Here's how the part is built. I have some questions about the finished solid (model axes, mm). Round coordinates to 2 decimals unless told otherwise and drop trailing zeros. Order: outer loops, then holes, each group sorted by start corner. A loop starts at its lowest first (then second) coordinate and runs counter-clockwise, first axis right, second up.
```python
from build123d import *

# Parameters (mm, degrees)
F0_W     = 95
F0_H     = 25
F1_DEPTH = 8
F2_SIZE  = 2.5
F4_D     = 5.5
F4_DEPTH = 10
F4_TIP   = 1.6523667023
F6_D     = 6.5
F6_DEPTH = 10
F6_TIP   = 1.9527970118
F7_D     = 6.8


with BuildPart() as f1:
    # F0 (on Front) → F1 (new body)
    with BuildSketch(Plane.XZ):
        Rectangle(F0_W, F0_H)
    extrude(amount=F1_DEPTH)

    # F2
    f2_edges = [f1.edges().sort_by_distance(p)[0] for p in [
        (47.5, -4, 12.5),
        (47.5, -4, -12.5),
        (-47.5, -4, 12.5),
        (-47.5, -4, -12.5),
    ]]
    chamfer(f2_edges, length=F2_SIZE)

    # F4
    with Locations(Plane.XZ.offset(8)):
        with Locations((-41, 7.5), (-41, -7.5), (41, -7.5), (41, 7.5)):
            Hole(F4_D / 2, depth=F4_DEPTH)
            with Locations((0, 0, -(F4_DEPTH + F4_TIP / 2))):  # 118° drill point
                Cone(0, F4_D / 2, F4_TIP, mode=Mode.SUBTRACT)

    # F6
    with Locations(Plane.XZ.offset(8)):
        with Locations((-29, 5), (29, 5)):
            Hole(F6_D / 2, depth=F6_DEPTH)
            with Locations((0, 0, -(F6_DEPTH + F6_TIP / 2))):  # 118° drill point
                Cone(0, F6_D / 2, F6_TIP, mode=Mode.SUBTRACT)

    # F7 (through all)
    with Locations(Plane.XZ.offset(8)):
        with Locations((0, 0)):
            Hole(F7_D / 2)


solid = f1.part
```
1. If we mould it in two halves opening along Z, with no side actions, what happens to faces 1 (the flat face through (-1, -4, 12.5)), 2 (the cylindrical face through (25.9, -3.94, 5.98)), 3 (the flat face through (-1, -8, -5))? For each: released by +Z, released by -Z, zero draft, split by the parting line, or undercut.
Evaluation:
face 1: released by +Z
face 2: undercut
face 3: zero draft
2. I'm going to push a flat-ended pin straight in: P1, Ø5, axis at x = -41, z = -7.5, coming from the -Y side. Where does the tip first touch, or does it pass through?
Evaluation:
P1: passes through
3. If we section it at D-D, the plane x = 41: Write out the boundary of the cut face in (y, z), and give its area (3 significant figures).
Evaluation:
outline: (-8, -12.5) - (0, -12.5) - (0, -10.25) - (-8, -10.25) - close; (-8, -4.75) - (0, -4.75) - (0, 4.75) - (-8, 4.75) - close; (-8, 10.25) - (0, 10.25) - (0, 12.5) - (-8, 12.5) - close
area: 112 mm2
4. If we section it at A-A, the plane x = 0: Write out the boundary of the cut face in (y, z), and give its area (3 significant figures).
Evaluation:
outline: (-8, -12.5) - (0, -12.5) - (0, -3.4) - (-8, -3.4) - close; (-8, 3.4) - (0, 3.4) - (0, 12.5) - (-8, 12.5) - close
area: 146 mm2
5. If we section it at C-C, the plane y = -2.5: Write out the boundary of the cut face in (x, z), and give its area (3 significant figures).
Evaluation:
outline: (-47.5, -10) - (-45, -12.5) - (45, -12.5) - (47.5, -10) - (47.5, 10) - (45, 12.5) - (-45, 12.5) - (-47.5, 10) - close; hole circle Ø5.5 at (-41, -7.5); hole circle Ø5.5 at (-41, 7.5); hole circle Ø6.5 at (-29, 5); hole circle Ø6.8 at (0, 0); hole circle Ø6.5 at (29, 5); hole circle Ø5.5 at (41, -7.5); hole circle Ø5.5 at (41, 7.5)
area: 2,160 mm2
6. I need wall thicknesses on probe 1 along Z at (x, y) = (41, -5); probe 2 along Z at (x, y) = (29, -4.75); probe 3 along Z at (x, y) = (0, -4.5). Which ranges of each line are inside material? Lowest first, please.
Evaluation:
probe 1: z = -12.5 to -10.25, -4.75 to 4.75, 10.25 to 12.5
probe 2: z = -12.5 to 1.75, 8.25 to 12.5
probe 3: z = -12.5 to -3.4, 3.4 to 12.5
7. If we section it at B-B, the plane z = 0: Write out the boundary of the cut face in (x, y).
Evaluation:
outline: (-47.5, -8) - (-3.4, -8) - (-3.4, 0) - (-47.5, 0) - close; (3.4, -8) - (47.5, -8) - (47.5, 0) - (3.4, 0) - close
